```python
from build123d import *

# Parameters (mm, degrees)
EXTRUDE_1_DEPTH     = 3
SKETCH_2_R          = 1.6
CUT_EXTRUDE_1_DEPTH = 66.261014396


with BuildPart() as part:
    # 草图1 → 凸台-拉伸1 (new body)
    with BuildSketch(Plane.XY):
        Polygon((0, 0), (15, 0), (35, -20), (35, -35), (15, -55), (0, -55), (-20, -35), (-20, -20), align=None)
    extrude(amount=EXTRUDE_1_DEPTH)

    # 草图2 → 切除-拉伸1 (cut, through all)
    with BuildSketch(Plane(origin=(0, 0, 0), x_dir=(-1, 0, 0), z_dir=(0, 0, -1))):
        with Locations((-11.25, -5)):
            Circle(SKETCH_2_R)
        with Locations((-30, -31.25)):
            Circle(SKETCH_2_R)
        with Locations(Location((-30, -23.75, 0), (0, 0, 180))):
            Circle(SKETCH_2_R)
        with Locations(Location((-3.75, -5, 0), (0, 0, 180))):
            Circle(SKETCH_2_R)
        with Locations((-3.75, -15)):
            Circle(SKETCH_2_R)
        with Locations(Location((-11.25, -15, 0), (0, 0, 180))):
            Circle(SKETCH_2_R)
        with Locations((-20, -23.75)):
            Circle(SKETCH_2_R)
        with Locations(Location((-20, -31.25, 0), (0, 0, 180))):
            Circle(SKETCH_2_R)
        with Locations((5, -31.25)):
            Circle(SKETCH_2_R)
        with Locations(Location((5, -23.75, 0), (0, 0, 180))):
            Circle(SKETCH_2_R)
        with Locations((15, -23.75)):
            Circle(SKETCH_2_R)
        with Locations(Location((15, -31.25, 0), (0, 0, 180))):
            Circle(SKETCH_2_R)
        with Locations((-11.25, -40)):
            Circle(SKETCH_2_R)
        with Locations(Location((-3.75, -40, 0), (0, 0, 180))):
            Circle(SKETCH_2_R)
        with Locations((-3.75, -50)):
            Circle(SKETCH_2_R)
        with Locations(Location((-11.25, -50, 0), (0, 0, 180))):
            Circle(SKETCH_2_R)
    extrude(amount=-CUT_EXTRUDE_1_DEPTH, mode=Mode.SUBTRACT)


solid = part.part
```
For this review, take the finished solid that the model builds, in its own axes (mm). Round coordinates to 2 decimals unless told otherwise and drop trailing zeros. Write each loop counter-clockwise with the first axis right and the second up, starting at its lowest first coordinate (ties: lowest second). Pieces come first, ordered by that corner, then holes. Notation, with made-up numbers: (71.25, 89) - (117.25, 89) arc R32 cw to (117.25, 119) - close; hole circle Ø2 at (-12.75, -19.75). An arc over 180 degrees is marked (long way). Answer as a JSON object with one key per item and string values.
1. We need section D-D on z = 1.95. Count the separate pieces of the cut face and the enclosed holes in it, then the cut area to 3 significant figures.
Response values:
{"separate pieces": "1", "enclosed holes": "16", "area": "2,100 mm2"}
2. We need section B-B on y = -50. Give the boundary of the cut face in (x, z).
Response values:
{"outline": "(-5, 0) - (2.15, 0) - (2.15, 3) - (-5, 3) - close; (5.35, 0) - (9.65, 0) - (9.65, 3) - (5.35, 3) - close; (12.85, 0) - (20, 0) - (20, 3) - (12.85, 3) - close"}
3. We need section C-C on y = -23.75. Give the boundary of the cut face in (x, z), then the cut area to 3 significant figures.
Response values:
{"outline": "(-20, 0) - (-16.6, 0) - (-16.6, 3) - (-20, 3) - close; (-13.4, 0) - (-6.6, 0) - (-6.6, 3) - (-13.4, 3) - close; (-3.4, 0) - (18.4, 0) - (18.4, 3) - (-3.4, 3) - close; (21.6, 0) - (28.4, 0) - (28.4, 3) - (21.6, 3) - close; (31.6, 0) - (35, 0) - (35, 3) - (31.6, 3) - close", "area": "127 mm2"}
4. Draft analysis for pull direction Y (two halves, no side actions). For faces 1 (the face through (-20, -28, 1)), 2 (the face through (9.65, -15.07, 1.48)), 3 (the face through (25, -45, 1)), 4 (the face through (25, -10, 1)), state which applies: +Y half, -Y half, draft (parallel to the pull), parting line (faces both ways), or undercut.
Response values:
{"face 1": "draft", "face 2": "undercut", "face 3": "-Y half", "face 4": "+Y half"}
5. We need section A-A on x = 3.75. Give the boundary of the cut face in (y, z).
Response values:
{"outline": "(-55, 0) - (-51.6, 0) - (-51.6, 3) - (-55, 3) - close; (-48.4, 0) - (-41.6, 0) - (-41.6, 3) - (-48.4, 3) - close; (-38.4, 0) - (-16.6, 0) - (-16.6, 3) - (-38.4, 3) - close; (-13.4, 0) - (-6.6, 0) - (-6.6, 3) - (-13.4, 3) - close; (-3.4, 0) - (0, 0) - (0, 3) - (-3.4, 3) - close"}
6. To check wall thickness, follow line 1 along Y through (x, z) = (11.25, 1.65); line 2 along Y through (x, z) = (29, 0.75); line 3 along X through (y, z) = (-41, 0.7). State the ranges of each line that lie inside material, in increasing order.
Response values:
{"line 1": "y = -55 to -51.6, -48.4 to -41.6, -38.4 to -16.6, -13.4 to -6.6, -3.4 to 0", "line 2": "y = -41 to -32.5, -30 to -25, -22.5 to -14", "line 3": "x = -14 to 2.5, 5 to 10, 12.5 to 29"}
